Input: part model. Units: mm. Frame: model coordinates. A direction names the side the tool comes from. Coordinates: 2 decimals unless noted, no trailing zeros. Write each loop counter-clockwise with the first axis right and the second up, starting at its lowest first coordinate (ties: lowest second). Pieces come first, ordered by that corner, then holes. Notation, with made-up numbers: M 28.5,4.5 L 53.5,4.5 A20 ccw 53.5,17.5 Z; hole C 72.5,79.5 d2. An arc over 180 degrees is marked long. Use one line per item in the form item = value.
from build123d import *

# Parameters (mm, degrees)
F0_R     = 27.4243717003
F1_DEPTH = 35
F2_DEPTH = 7.35
F0_R_2   = 0.735
F0_R_3   = 4.94
F3_DEPTH = 2.2
F4_DEPTH = 2.30452
F5_R     = 4.94
F6_DEPTH = 31.99051


with BuildPart() as f1:
    # F0 (on Top) → F1 (new body)
    with BuildSketch(Plane.XY):
        Circle(F0_R)
        with BuildLine():
            ThreePointArc((22.4924149425, 12.9118354642), (24.1955551249, 9.3380585348), (25.3349236359, 5.546698961))
            ThreePointArc((25.3349236359, 5.546698961), (25.7845444937, 2.789532264), (25.935, 0))
            ThreePointArc((25.935, 0), (24.9905557449, -6.935153103), (22.2260084009, -13.3652076513))
            ThreePointArc((22.2260084009, -13.3652076513), (19.0060906975, -17.6463237361), (14.9753258207, -21.1746036932))
            ThreePointArc((14.9753258207, -21.1746036932), (2.1917464406, -25.8422226703), (-11.1953286546, -23.3942052935))
            ThreePointArc((-11.1953286546, -23.3942052935), (-15.3006955677, -20.9407005648), (-18.8857364827, -17.775071941))
            ThreePointArc((-18.8857364827, -17.775071941), (-24.5544366053, -8.3488842366), (-25.8064478461, 2.5790452823))
            ThreePointArc((-25.8064478461, 2.5790452823), (-24.7694228602, 7.6876469855), (-22.7317421539, 12.4856767398))
            ThreePointArc((-22.7317421539, 12.4856767398), (-14.2591316257, 21.6633651652), (-2.4791175308, 25.8162391))
            ThreePointArc((-2.4791175308, 25.8162391), (0.1109366843, 25.9347627337), (2.6998821615, 25.7940857817))
            ThreePointArc((2.6998821615, 25.7940857817), (14.1474750982, 21.7364480388), (22.4924149425, 12.9118354642))
        make_face(mode=Mode.SUBTRACT)
    extrude(amount=F1_DEPTH)

    # F0 (on Top) → F2 (join)
    with BuildSketch(Plane.XY):
        with BuildLine():
            Line((22.2260084009, -13.3652076513), (7.4958561826, -4.3467648993))
            ThreePointArc((7.4958561826, -4.3467648993), (5.751506041, -6.4809261113), (3.4251739378, -7.959296985))
            Line((3.4251739378, -7.959296985), (14.9753258207, -21.1746036932))
            ThreePointArc((14.9753258207, -21.1746036932), (19.0060906975, -17.6463237361), (22.2260084009, -13.3652076513))
        make_face()
        with BuildLine():
            ThreePointArc((7.0672034825, 5.0136673141), (7.9748170172, 3.3888816064), (8.5145365353, 1.6077601153))
            Line((8.5145365353, 1.6077601153), (25.3349236359, 5.546698961))
            ThreePointArc((25.3349236359, 5.546698961), (24.1955551249, 9.3380585348), (22.4924149425, 12.9118354642))
            Line((22.4924149425, 12.9118354642), (7.0672034825, 5.0136673141))
        make_face()
        with BuildLine():
            ThreePointArc((-1.7975824717, 8.4764923322), (0.4672047175, 8.6523953187), (2.6998821615, 8.2336420443))
            Line((2.6998821615, 8.2336420443), (2.6998821615, 25.7940857817))
            ThreePointArc((2.6998821615, 25.7940857817), (0.1109366843, 25.9347627337), (-2.4791175308, 25.8162391))
            Line((-2.4791175308, 25.8162391), (-1.7975824717, 8.4764923322))
        make_face()
        with BuildLine():
            ThreePointArc((-8.0730394743, -3.1477386559), (-8.5412222171, 1.4593656284), (-6.569904314, 5.6496532907))
            Line((-6.569904314, 5.6496532907), (-22.7317421539, 12.4856767398))
            ThreePointArc((-22.7317421539, 12.4856767398), (-24.7694228602, 7.6876469855), (-25.8064478461, 2.5790452823))
            Line((-25.8064478461, 2.5790452823), (-8.0730394743, -3.1477386559))
        make_face()
        with BuildLine():
            Line((-11.1953286546, -23.3942052935), (-3.3863183591, -7.9759057774))
            ThreePointArc((-3.3863183591, -7.9759057774), (-4.6322458356, -7.3228767242), (-5.7560910789, -6.4768542126))
            Line((-5.7560910789, -6.4768542126), (-18.8857364827, -17.775071941))
            ThreePointArc((-18.8857364827, -17.775071941), (-15.3006955677, -20.9407005648), (-11.1953286546, -23.3942052935))
        make_face()
    extrude(amount=F2_DEPTH)

    # F0 (on Top) → F3 (join)
    with BuildSketch(Plane.XY):
        with BuildLine():
            ThreePointArc((7.4958561826, -4.3467648993), (8.3676107349, -2.2506255995), (8.665, 0))
            ThreePointArc((8.665, 0), (8.6273021298, 0.807392693), (8.5145365353, 1.6077601153))
            ThreePointArc((8.5145365353, 1.6077601153), (7.9748170172, 3.3888816064), (7.0672034825, 5.0136673141))
            ThreePointArc((7.0672034825, 5.0136673141), (5.1420861341, 6.9743225614), (2.6998821615, 8.2336420443))
            ThreePointArc((2.6998821615, 8.2336420443), (0.4672047175, 8.6523953187), (-1.7975824717, 8.4764923322))
            ThreePointArc((-1.7975824717, 8.4764923322), (-4.4160461409, 7.4552505981), (-6.569904314, 5.6496532907))
            ThreePointArc((-6.569904314, 5.6496532907), (-8.5412222171, 1.4593656284), (-8.0730394743, -3.1477386559))
            ThreePointArc((-8.0730394743, -3.1477386559), (-7.1120999404, -4.9497736754), (-5.7560910789, -6.4768542126))
            ThreePointArc((-5.7560910789, -6.4768542126), (-4.6322458356, -7.3228767242), (-3.3863183591, -7.9759057774))
            ThreePointArc((-3.3863183591, -7.9759057774), (0.0211282274, -8.664974241), (3.4251739378, -7.959296985))
            ThreePointArc((3.4251739378, -7.959296985), (5.751506041, -6.4809261113), (7.4958561826, -4.3467648993))
        make_face()
        with Locations((-5.658719223, -3.3904951997)):
            Circle(F0_R_2, mode=Mode.SUBTRACT)
        with Locations((5.5777155794, -3.3904951997)):
            Circle(F0_R_2, mode=Mode.SUBTRACT)
        with Locations((-5.5862264708, 4.1487901472)):
            Circle(F0_R_2, mode=Mode.SUBTRACT)
        Circle(F0_R_3, mode=Mode.SUBTRACT)
        with Locations((5.5777155794, 4.1487901472)):
            Circle(F0_R_2, mode=Mode.SUBTRACT)
    extrude(amount=F3_DEPTH)

    # F0 (on Top) → F4 (join)
    with BuildSketch(Plane.XY):
        Circle(F0_R_3)
    extrude(amount=F4_DEPTH)

    # F5 (on face) → F6 (join)
    with BuildSketch(Plane.XY.offset(2.30452)):
        Circle(F5_R)
        with BuildLine():
            Line((1.0092968587, 1.861386816), (1.0092968587, -1.861386816))
            Line((1.0092968587, -1.861386816), (0.9870916385, -1.861386816))
            ThreePointArc((0.9870916385, -1.861386816), (0, -2.8484784545), (-0.9870916385, -1.861386816))
            Line((-0.9870916385, -1.861386816), (-1.0092968587, -1.861386816))
            Line((-1.0092968587, -1.861386816), (-1.0092968587, 1.861386816))
            Line((-1.0092968587, 1.861386816), (-1.0026240675, 1.861386816))
            ThreePointArc((-1.0026240675, 1.861386816), (0, 2.8640108835), (1.0026240675, 1.861386816))
            Line((1.0026240675, 1.861386816), (1.0092968587, 1.861386816))
        make_face(mode=Mode.SUBTRACT)
    extrude(amount=F6_DEPTH)


solid = f1.part
(1) Section query C-C on y = 23.5. Return the cut outline in (x, z).
Computed:
outline = M -14.14,0 L -10.97,0 L -10.97,35 L -14.14,35 Z; M -2.39,0 L 2.7,0 L 2.7,7.35 L -2.39,7.35 Z; M 10.97,0 L 14.14,0 L 14.14,35 L 10.97,35 Z
(2) First-contact query: pin 1 Ø14 at (x, y) = (2.5, -2) entering from +Z (3 decimals); pin 2 Ø5.5 at (x, y) = (-0.5, 20.5) entering from +Z; pin 3 Ø3 at (x, z) = (-9.5, 31) entering from -Y; pin 4 Ø0.9 at (x, y) = (5.58, 4.15) entering from +Z. Flat tips, straight axial feed; report the tip coordinate or a pass-through.
Computed:
pin_1 = 34.295
pin_2 = 7.35
pin_3 = -26.23
pin_4 = through
(3) Section query B-B on x = 0. Return the cut outline in (y, z) (3 decimals).
Computed:
outline = M -27.424,0 L -25.935,0 L -25.935,35 L -27.424,35 Z; M -8.665,0 L 27.424,0 L 27.424,35 L 25.935,35 L 25.935,7.35 L 8.665,7.35 L 8.665,2.2 L 4.94,2.2 L 4.94,34.295 L 2.864,34.295 L 2.864,2.305 L -2.848,2.305 L -2.848,34.295 L -4.94,34.295 L -4.94,2.2 L -8.665,2.2 Z
(4) Pull-direction query (Y, two-part tool) for faces 3 (the cylindrical face through (26.158, 8.238, 17.255)), 4 (the flat face through (24.2, -10, 35)), 5 (the cylindrical face through (-4.907, 3.867, 1.085)); classes: pulls with the +Y half, pulls with the -Y half, needs draft (parallel to the pull), parting line crosses it, or undercut.
Computed:
face_3 = parting line crosses it
face_4 = needs draft
face_5 = undercut
(5) Section query A-A on z = 24. Return the cut outline in (x, y) (3 decimals), plus the area to 3 significant figures.
Computed:
outline = C 0,0 d54.849; C 0,0 d9.88; hole C 0,0 d51.87; hole M -1.009,-1.861 L -0.987,-1.861 A0.987 ccw 0.987,-1.861 L 1.009,-1.861 L 1.009,1.861 L 1.003,1.861 A1.003 ccw -1.003,1.861 L -1.009,1.861 Z
area = 316 mm^2
(6) Line query: probe 1 along X at (y, z) = (-1, 27); probe 2 along Y at (x, z) = (-9, 3); probe 3 along X at (y, z) = (10, 11). Output: solid intervals per line, ascending.
Computed:
probe_1 = -27.41 to -25.92, -4.84 to -1.01, 1.01 to 4.84, 25.92 to 27.41
probe_2 = -25.91 to -24.32, -19.06 to -9.27, -2.85 to 6.68, 24.32 to 25.91
probe_3 = -25.54 to -23.93, 23.93 to 25.54
(7) Section query D-D on x = 20.5. Return the cut outline in (y, z), plus the area to 3 significant figures.
Computed:
outline = M -18.22,0 L -12.31,0 L -12.31,7.35 L -15.89,7.35 L -15.89,35 L -18.22,35 Z; M 4.41,0 L 11.89,0 L 11.89,7.35 L 4.41,7.35 Z; M 15.89,0 L 18.22,0 L 18.22,35 L 15.89,35 Z
area = 244 mm^2
(8) Set-up query: faces 1 (the flat face through (-1.2, 0.1, 34.295)), 2 (the flat face through (2.7, 17, 4)). Return all of +Z, -Z, +X, -X, +Y, -Y with unobstructed straight access to the full face (end or side cutting, diameter ignored); none if empty.
Computed:
face_1 = +Z
face_2 = +Z, -Z
